```python
from build123d import *

# Parameters (mm, degrees)
BOSS_EXTRUDE1_DEPTH = 3
CUT_EXTRUDE1_REACH  = 5


with BuildPart() as part:
    # Sketch1 → Boss-Extrude1 (new body)
    with BuildSketch(Plane(origin=(0, 0, 0), x_dir=(1, 0, 0), z_dir=(0, 1, 0))):
        with BuildLine():
            Line((1.35, 14.954385483), (-1.35, 14.954385483))
            Line((-1.35, 14.954385483), (-1.35, 19.954385483))
            ThreePointArc((-1.35, 19.954385483), (-14.142135624, 14.142135624), (-19.954385483, 1.35))
            Line((-19.954385483, 1.35), (-14.954385483, 1.35))
            Line((-14.954385483, 1.35), (-14.954385483, -1.35))
            Line((-14.954385483, -1.35), (-19.954385483, -1.35))
            ThreePointArc((-19.954385483, -1.35), (-14.142135624, -14.142135624), (-1.35, -19.954385483))
            Line((-1.35, -19.954385483), (-1.35, -14.954385483))
            Line((-1.35, -14.954385483), (1.35, -14.954385483))
            Line((1.35, -14.954385483), (1.35, -19.954385483))
            ThreePointArc((1.35, -19.954385483), (14.142135624, -14.142135624), (19.954385483, -1.35))
            Line((19.954385483, -1.35), (14.954385483, -1.35))
            Line((14.954385483, -1.35), (14.954385483, 1.35))
            Line((14.954385483, 1.35), (19.954385483, 1.35))
            ThreePointArc((19.954385483, 1.35), (14.142135624, 14.142135624), (1.35, 19.954385483))
            Line((1.35, 19.954385483), (1.35, 14.954385483))
        make_face()
    extrude(amount=BOSS_EXTRUDE1_DEPTH)

    # Sketch3 → Cut-Extrude1 (cut, up to next)
    with BuildSketch(Plane(origin=(0, 3, 0), x_dir=(1, 0, 0), z_dir=(0, 1, 0)), mode=Mode.PRIVATE) as cut_extrude1_sk1:
        Polygon((1.45, 1.45), (10, 1.45), (10, -1.45), (1.45, -1.45), (1.45, -10), (-1.45, -10), (-1.45, -1.45), (-10, -1.45), (-10, 1.45), (-1.45, 1.45), (-1.45, 10), (1.45, 10), align=None)
    cut_extrude1_tool1 = extrude(cut_extrude1_sk1.sketch, amount=-CUT_EXTRUDE1_REACH, mode=Mode.PRIVATE) & part.part
    add(cut_extrude1_tool1.solids().sort_by_distance((0, 3, 0))[0], mode=Mode.SUBTRACT)


solid = part.part
```
Geometry check sheet. Reference: the model listing, model coordinates, mm. A direction names the side the tool comes from. Give positions to 0.01 mm unless a question says otherwise; leave off trailing zeros. Write each loop counter-clockwise with the first axis right and the second up, starting at its lowest first coordinate (ties: lowest second). Pieces come first, ordered by that corner, then holes.
1) Section check D-D, the plane z = -11. Record the boundary of the cut face in (x, y).
2) Section check C-C, the plane x = -5. Record the boundary of the cut face in (y, z).
3) Section check B-B, the plane y = 2.2. Record the boundary of the cut face in (x, z).
4) Section check A-A, the plane z = 16. Record the boundary of the cut face in (x, y), and give its area (3 significant figures).
5) Gauge pin test, flat ends, axial feed: pin 1 (1.5 mm diameter, centred on y = 1, z = -6, fed in from +X); pin 2 (1.5 mm diameter, centred on x = -5.5, y = 1.5, fed in from +Z); pin 3 (1.5 mm diameter, centred on x = 6.5, y = 1.5, fed in from +Z); pin 4 (1.5 mm diameter, centred on x = -0.5, z = -16, fed in from -Y). Record the tip position at first contact, or that the pin passes through.
6) Access from +Z, -Z, +X, -X, +Y, -Y to the whole of each face (thin tool, end or side, straight path). Record for faces 5 (the flat face through (-1.35, 1, 17)), 6 (the flat face through (-1.45, 2, -6)), 7 (the flat face through (0, 1, -14.954)).
7) Material ranges on L1, parallel to Z at x = -9.5, y = 0.45; L2, parallel to X at y = 2.15, z = -6.5; L3, parallel to Z at x = 17.5, y = 0.4, recorded low to high.
8) Release check for a two-part mould opening along X. For faces 1 (the flat face through (17, 1, 1.35)), 2 (the cylindrical face through (13.999, 1.479, 14.284)), 3 (the flat face through (-1.35, 1, -17)), 4 (the cylindrical face through (-14.284, 1.479, 13.999)) record: pulls with the +X half, pulls with the -X half, needs draft (parallel to the pull), parting line crosses it, or undercut.
Computed:
1. outline: (-16.7, 0) - (16.7, 0) - (16.7, 3) - (-16.7, 3) - close
2. outline: (0, -19.36) - (3, -19.36) - (3, -1.45) - (0, -1.45) - close; (0, 1.45) - (3, 1.45) - (3, 19.36) - (0, 19.36) - close
3. outline: (-19.95, -1.35) arc R20 ccw to (-1.35, -19.95) - (-1.35, -14.95) - (1.35, -14.95) - (1.35, -19.95) arc R20 ccw to (19.95, -1.35) - (14.95, -1.35) - (14.95, 1.35) - (19.95, 1.35) arc R20 ccw to (1.35, 19.95) - (1.35, 14.95) - (-1.35, 14.95) - (-1.35, 19.95) arc R20 ccw to (-19.95, 1.35) - (-14.95, 1.35) - (-14.95, -1.35) - close; hole (-10, -1.45) - (-1.45, -1.45) - (-1.45, -10) - (1.45, -10) - (1.45, -1.45) - (10, -1.45) - (10, 1.45) - (1.45, 1.45) - (1.45, 10) - (-1.45, 10) - (-1.45, 1.45) - (-10, 1.45) - close
4. outline: (-12, 0) - (-1.35, 0) - (-1.35, 3) - (-12, 3) - close; (1.35, 0) - (12, 0) - (12, 3) - (1.35, 3) - close
4. area: 63.9 mm2
5. pin 1: stops at x = 19.3
5. pin 2: stops at z = 19.43
5. pin 3: stops at z = 19.16
5. pin 4: passes through
6. face 5: +Z, +Y, -Y
6. face 6: +Y, -Y
6. face 7: -Z, +Y, -Y
7. L1: z = -17.6 to -1.45, 1.45 to 17.6
7. L2: x = -18.91 to -1.45, 1.45 to 18.91
7. L3: z = -9.68 to -1.35, 1.35 to 9.68
8. face 1: needs draft
8. face 2: pulls with the +X half
8. face 3: undercut
8. face 4: pulls with the -X half
